Print and shaded views of the part. All mm, measured from the part's lowest x, y and z. A direction names the side the tool comes from. Coordinates: 2 decimals unless noted, no trailing zeros. Order: outer loops, then holes, each group sorted by start corner. A loop starts at its lowest first (then second) coordinate and runs counter-clockwise, first axis right, second up. Notation, with made-up numbers: (37.25, 36) -> (50.25, 36) arc R16 cw to (50.25, 56) -> close; hole circle Ø6 at (-33.75, -31.5). An arc over 180 degrees is marked (long way). Return JSON: item names as keys, results as strings. Group by question number.
1) Probe line 1 (Z direction, x = 3.25, y = 7.25); line 2 (Z direction, x = 6.5, y = 14); line 3 (Y direction, x = 8.25, z = 16.25). List the from-to ranges inside material, lowest first.
2) Cut at D-D (y = 13). Write the cut outline in (x, z), and give its area (3 significant figures).
3) Which spindle directions (+Z, -Z, +X, -X, +Y, -Y) get a long thin tool onto all of the face, cutting with end or side? Do the marked faces 1, 2 and 3. Say none if no direction does.
4) Cut at A-A (y = 8.1). Write the cut outline in (x, z).
5) Flat gauge pins, fed straight in: pin 1 (5 mm diameter, centred on y = 6.5, z = 6, fed in from -X); pin 2 (8 mm diameter, centred on x = 3.5, z = 21, fed in from -Y); pin 3 (1 mm diameter, centred on y = 4, z = 17, fed in from +X). Where does each tip first touch, or does it go through?
6) Cut at C-C (z = 18.5). Write the cut outline in (x, y), and give its area (3 significant figures).
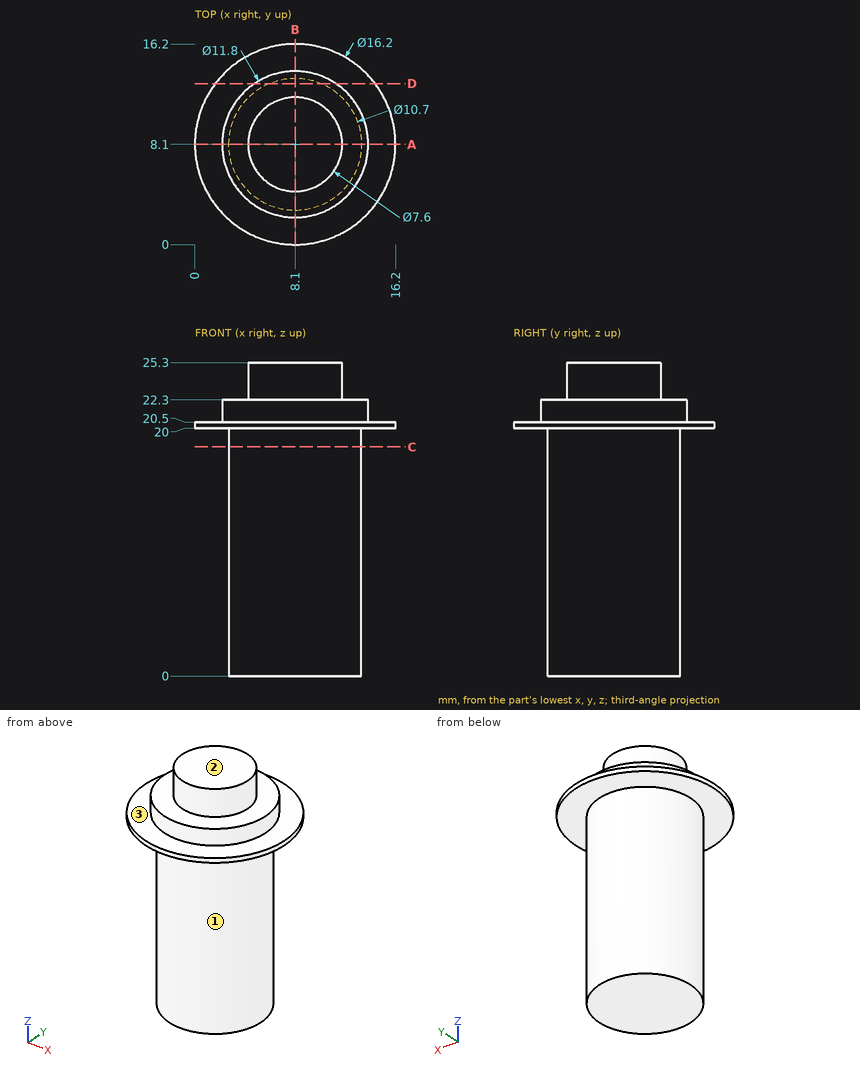
Answers below:
{
 "1": {"line 1": "z = 0 to 22.3", "line 2": "z = 20 to 20.5", "line 3": "y = 2.75 to 13.45"},
 "2": {"outline": "(1.65, 20) -> (5.95, 20) -> (5.95, 0) -> (10.25, 0) -> (10.25, 20) -> (14.55, 20) -> (14.55, 20.5) -> (11.39, 20.5) -> (11.39, 22.3) -> (4.81, 22.3) -> (4.81, 20.5) -> (1.65, 20.5) -> close", "area": "104 mm^2"},
 "3": {"face 1": "-Z", "face 2": "+Z, +X, -X, +Y, -Y", "face 3": "+Z"},
 "4": {"outline": "(0, 20) -> (2.75, 20) -> (2.75, 0) -> (13.45, 0) -> (13.45, 20) -> (16.2, 20) -> (16.2, 20.5) -> (14, 20.5) -> (14, 22.3) -> (11.9, 22.3) -> (11.9, 25.3) -> (4.3, 25.3) -> (4.3, 22.3) -> (2.2, 22.3) -> (2.2, 20.5) -> (0, 20.5) -> close"},
 "5": {"pin 1": "stops at x = 2.75", "pin 2": "stops at y = 0.02", "pin 3": "stops at x = 12.06"},
 "6": {"outline": "circle Ø10.7 at (8.1, 8.1)", "area": "89.9 mm^2"}
}
